Build history of the part. All positions in model axes, mm. Face numbers are marked on the shaded views. A direction names the side the tool comes from. Round coordinates to 2 decimals unless told otherwise and drop trailing zeros. Loops run counter-clockwise (first coordinate to the right, second up) from the corner with the lowest first, then second, coordinate; pieces in that order, holes last. Notation, with made-up numbers: M 87,1.25 L 111,1.25 A30 ccw 111,32.25 Z; hole C 47,64 d10. An arc over 180 degrees is marked long. Use one line per item in the form item = value. Start each with the question number.
```python
from build123d import *

# Parameters (mm, degrees)
SKETCH007_W     = 80
SKETCH007_H     = 80
PAD005_DEPTH    = 100
POCKET001_DEPTH = 80.001
POCKET002_DEPTH = 80.001
SKETCH011_W     = 37
SKETCH011_H     = 1660.928571
POCKET003_DEPTH = 37
SKETCH012_R     = 12
POCKET004_DEPTH = 4
SKETCH013_R     = 2
POCKET005_DEPTH = 10.501
SKETCH014_R     = 3
POCKET006_DEPTH = 4.5
SKETCH016_W     = 16
SKETCH016_H     = 89.5
POCKET008_DEPTH = 14
SKETCH024_W     = 16
SKETCH024_H     = 89.5
POCKET015_DEPTH = 14
SKETCH018_R     = 3
POCKET010_DEPTH = 5
SKETCH022_R     = 1.3
POCKET013_DEPTH = 10
CHAMFER_SIZE    = 5


with BuildPart() as part:
    # Sketch007 → Pad005 (new body)
    with BuildSketch(Plane.XY):
        Rectangle(SKETCH007_W, SKETCH007_H)
    extrude(amount=PAD005_DEPTH)

    # Sketch008 (on Face2 of Pad005) → Pocket001 (cut, through all)
    with BuildSketch(Plane.XZ.offset(40)):
        Polygon((-40, 0), (0, 100), (-40, 100), align=None)
        Polygon((-30, 8), (-5, 8), (-5, 33), (-20, 33), align=None)
    extrude(amount=-POCKET001_DEPTH, mode=Mode.SUBTRACT)

    # Sketch009 (on Face4 of Pocket001) → Pocket002 (cut, through all)
    with BuildSketch(Plane.YZ.offset(40)):
        Polygon((-36.5, 100), (-40, 0), (-40, 100), align=None)
        Polygon((40, 0), (36.5, 100), (40, 100), align=None)
    extrude(amount=-POCKET002_DEPTH, mode=Mode.SUBTRACT)

    # Sketch011 (on Face4 of Pocket002) → Pocket003 (cut)
    with BuildSketch(Plane.YZ.offset(40)):
        with Locations((0, 840.964285)):
            Rectangle(SKETCH011_W, SKETCH011_H)
    extrude(amount=-POCKET003_DEPTH, mode=Mode.SUBTRACT)

    # Sketch012 (on Face12 of Pocket003) → Pocket004 (cut)
    with BuildSketch(Plane.XY.offset(10.5)):
        with Locations((21.5, 0)):
            Circle(SKETCH012_R)
    extrude(amount=-POCKET004_DEPTH, mode=Mode.SUBTRACT)

    # Sketch013 (on Face12 of Pocket004) → Pocket005 (cut, through all)
    with BuildSketch(Plane.XY.offset(10.5)):
        with Locations((8, 13.5)):
            Circle(SKETCH013_R)
        with Locations((35, 13.5)):
            Circle(SKETCH013_R)
        with Locations((35, -13.5)):
            Circle(SKETCH013_R)
        with Locations((8, -13.5)):
            Circle(SKETCH013_R)
    extrude(amount=-POCKET005_DEPTH, mode=Mode.SUBTRACT)

    # Sketch014 (on Face1 of Pocket005) → Pocket006 (cut)
    with BuildSketch(Plane(origin=(0, 0, 0), x_dir=(1, 0, 0), z_dir=(0, 0, -1))):
        with Locations((8, 13.5)):
            Circle(SKETCH014_R)
        with Locations((35, 13.5)):
            Circle(SKETCH014_R)
        with Locations((35, -13.5)):
            Circle(SKETCH014_R)
        with Locations((8, -13.5)):
            Circle(SKETCH014_R)
    extrude(amount=-POCKET006_DEPTH, mode=Mode.SUBTRACT)

    # Sketch016 (on Face15 of Pocket006) → Pocket008 (cut)
    with BuildSketch(Plane.XZ.offset(-18.5)):
        with Locations((21.5, 55.25)):
            Rectangle(SKETCH016_W, SKETCH016_H)
    extrude(amount=-POCKET008_DEPTH, mode=Mode.SUBTRACT)

    # Sketch024 (on Face16 of Pocket008) → Pocket015 (cut)
    with BuildSketch(Plane(origin=(0, -18.5, 0), x_dir=(-1, 0, 0), z_dir=(0, 1, 0))):
        with Locations((-21.5, 55.25)):
            Rectangle(SKETCH024_W, SKETCH024_H)
    extrude(amount=-POCKET015_DEPTH, mode=Mode.SUBTRACT)

    # Sketch018 (on Face34 of Pocket015) → Pocket010 (cut)
    with BuildSketch(Plane.XY.offset(10.5)):
        with Locations((21.5, -25.5)):
            Circle(SKETCH018_R)
        with Locations((21.5, 25.5)):
            Circle(SKETCH018_R)
    extrude(amount=-POCKET010_DEPTH, mode=Mode.SUBTRACT)

    # Sketch022 (on Face10 of Pocket010) → Pocket013 (cut)
    with BuildSketch(Plane.XY.offset(100)):
        with Locations((6.75, 27.5)):
            Circle(SKETCH022_R)
        with Locations((34.75, 27.5)):
            Circle(SKETCH022_R)
        with Locations((6.75, -27.5)):
            Circle(SKETCH022_R)
        with Locations((34.75, -27.5)):
            Circle(SKETCH022_R)
    extrude(amount=-POCKET013_DEPTH, mode=Mode.SUBTRACT)

    # Chamfer
    chamfer_edges = [part.edges().sort_by_distance(p)[0] for p in [
        (29.5, -18.5, 55.25),
        (13.5, -18.5, 55.25),
        (13.5, 18.5, 55.25),
        (29.5, 18.5, 55.25),
    ]]
    chamfer(chamfer_edges, length=CHAMFER_SIZE)


solid = part.part
```
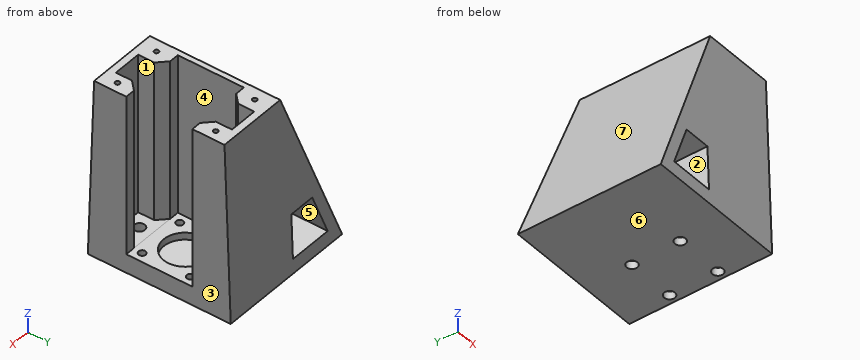
Q1. Saw through at A-A (y = 13.5). Give the cut face in (x, z), and give its area (3 significant figures).
Q2. Wall check: probe 1 along Y at (x, z) = (34.75, 96); probe 2 along X at (y, z) = (-21, 19); probe 3 along X at (y, z) = (19.5, 31.5). Give the ranges that are in metal, low to high.
Q3. Saw through at B-B (z = 50). Give the cut face in (x, y).
Q4. Saw through at C-C (x = -27). Give the cut face in (y, z), and give its area (3 significant figures).
Q5. Drop flat-ended pins along their axis: P1, Ø2, axis at x = 7, y = -27.5, coming from the +Z side; P2, Ø6.5, axis at x = 9, y = -14.5, coming from the -Z side; P3, Ø3, axis at x = 3, z = 16, coming from the -Y side; P4, Ø8, axis at y = 3, z = 88.5, coming from the -X side. Give the stop position or say it passes through.
Q6. Pull direction X, two halves, no side cores. Call the marked faces 5, 6 and 7: pulls with the +X half, pulls with the -X half, needs draft (parallel to the pull), parting line crosses it, or undercut.
Q7. Tool access for the marked faces 1, 2, 3 and 4: list every direction of +Z, -Z, +X, -X, +Y, -Y with a clear straight run to the whole face (end or side of a thin tool).
Q8. Saw through at D-D (z = 12.5). Give the cut face in (x, y), and give its area (3 significant figures).
Filled in:
q1.outline = M -40,0 L 5,0 L 5,4.5 L 6,4.5 L 6,10.5 L 3,10.5 L 3,100 L 0,100 Z; M 10,4.5 L 11,4.5 L 11,0 L 32,0 L 32,4.5 L 33,4.5 L 33,10.5 L 10,10.5 Z; M 37,4.5 L 38,4.5 L 38,0 L 40,0 L 40,10.5 L 37,10.5 Z; hole M -30,8 L -5,8 L -5,33 L -20,33 Z
q1.area = 2,090 mm²
q2.probe_1 = -36.64 to -28.8, -26.2 to -18.5, 18.5 to 26.2, 28.8 to 36.64
q2.probe_2 = -32.4 to -25.6, -5 to 11, 32 to 40
q2.probe_3 = -27.4 to -20.6, -5 to 9.5, 33.5 to 40
q3.outline = M -20,-38.25 L 40,-38.25 L 40,-18.5 L 34.5,-18.5 L 29.5,-23.5 L 29.5,-32.5 L 13.5,-32.5 L 13.5,-23.5 L 8.5,-18.5 L 3,-18.5 L 3,18.5 L 8.5,18.5 L 13.5,23.5 L 13.5,32.5 L 29.5,32.5 L 29.5,23.5 L 34.5,18.5 L 40,18.5 L 40,38.25 L -20,38.25 Z
q4.outline = M -40,0 L 40,0 L 39.72,8 L -39.72,8 Z; M -39.46,15.5 L 39.46,15.5 L 38.86,32.5 L -38.86,32.5 Z
q4.area = 1,970 mm²
q5.P1 = 90
q5.P2 = 0
q5.P3 = -39.49
q5.P4 = -6.2
q6.face_5 = undercut
q6.face_6 = needs draft
q6.face_7 = pulls with the -X half
q7.face_1 = +Z
q7.face_2 = +Y, -Y
q7.face_3 = +Z, -Z, +X, +Y, -Y
q7.face_4 = +Z, +X
q8.outline = M -35,-39.56 L -28.2,-39.56 L -28.2,39.56 L -35,39.56 Z; M -5,-39.56 L 40,-39.56 L 40,-18.5 L 34.5,-18.5 L 29.5,-23.5 L 29.5,-32.5 L 13.5,-32.5 L 13.5,-23.5 L 8.5,-18.5 L 3,-18.5 L 3,18.5 L 8.5,18.5 L 13.5,23.5 L 13.5,32.5 L 29.5,32.5 L 29.5,23.5 L 34.5,18.5 L 40,18.5 L 40,39.56 L -5,39.56 Z
q8.area = 2,230 mm²
